```python
from build123d import *

# Parameters (mm, degrees)
F2_DEPTH = 25


with BuildPart() as f2:
    # F1 (on Top) → F2 (new body)
    with BuildSketch(Plane.XY):
        with BuildLine():
            Line((-1.828092, -48.106283), (0, -48.106283))
            Line((0, -48.106283), (1.828092, -48.106283))
            Line((1.828092, -48.106283), (4.154787, -40.719498))
            ThreePointArc((4.154787, -40.719498), (6.403006, -40.426987), (8.63158, -40.010444))
            Line((8.63158, -40.010444), (13.12704, -46.316705))
            Line((13.12704, -46.316705), (14.865659, -45.751794))
            Line((14.865659, -45.751794), (16.604278, -45.186882))
            Line((16.604278, -45.186882), (16.534454, -37.442644))
            ThreePointArc((16.534454, -37.442644), (18.582246, -36.469712), (20.573027, -35.384888))
            Line((20.573027, -35.384888), (26.797206, -39.993326))
            Line((26.797206, -39.993326), (28.276164, -38.9188))
            Line((28.276164, -38.9188), (29.755121, -37.844275))
            Line((29.755121, -37.844275), (27.295614, -30.500643))
            ThreePointArc((27.295614, -30.500643), (28.942527, -28.942527), (30.500643, -27.295614))
            Line((30.500643, -27.295614), (37.844275, -29.755121))
            Line((37.844275, -29.755121), (38.9188, -28.276164))
            Line((38.9188, -28.276164), (39.993326, -26.797206))
            Line((39.993326, -26.797206), (35.384888, -20.573027))
            ThreePointArc((35.384888, -20.573027), (36.469712, -18.582246), (37.442644, -16.534454))
            Line((37.442644, -16.534454), (45.186882, -16.604278))
            Line((45.186882, -16.604278), (45.751794, -14.865659))
            Line((45.751794, -14.865659), (46.316705, -13.12704))
            Line((46.316705, -13.12704), (40.010444, -8.63158))
            ThreePointArc((40.010444, -8.63158), (40.426987, -6.403006), (40.719498, -4.154787))
            Line((40.719498, -4.154787), (48.106283, -1.828092))
            Line((48.106283, -1.828092), (48.106283, 0))
            Line((48.106283, 0), (48.106283, 1.828092))
            Line((48.106283, 1.828092), (40.719498, 4.154787))
            ThreePointArc((40.719498, 4.154787), (40.426987, 6.403006), (40.010444, 8.63158))
            Line((40.010444, 8.63158), (46.316705, 13.12704))
            Line((46.316705, 13.12704), (45.751794, 14.865659))
            Line((45.751794, 14.865659), (45.186882, 16.604278))
            Line((45.186882, 16.604278), (37.442644, 16.534454))
            ThreePointArc((37.442644, 16.534454), (36.469712, 18.582246), (35.384888, 20.573027))
            Line((35.384888, 20.573027), (39.993326, 26.797206))
            Line((39.993326, 26.797206), (38.9188, 28.276164))
            Line((38.9188, 28.276164), (37.844275, 29.755121))
            Line((37.844275, 29.755121), (30.500643, 27.295614))
            ThreePointArc((30.500643, 27.295614), (28.942527, 28.942527), (27.295614, 30.500643))
            Line((27.295614, 30.500643), (29.755121, 37.844275))
            Line((29.755121, 37.844275), (28.276164, 38.9188))
            Line((28.276164, 38.9188), (26.797206, 39.993326))
            Line((26.797206, 39.993326), (20.573027, 35.384888))
            ThreePointArc((20.573027, 35.384888), (18.582246, 36.469712), (16.534454, 37.442644))
            Line((16.534454, 37.442644), (16.604278, 45.186882))
            Line((16.604278, 45.186882), (14.865659, 45.751794))
            Line((14.865659, 45.751794), (13.12704, 46.316705))
            Line((13.12704, 46.316705), (8.63158, 40.010444))
            ThreePointArc((8.63158, 40.010444), (6.403006, 40.426987), (4.154787, 40.719498))
            Line((4.154787, 40.719498), (1.828092, 48.106283))
            Line((1.828092, 48.106283), (0, 48.106283))
            Line((0, 48.106283), (-1.828092, 48.106283))
            Line((-1.828092, 48.106283), (-4.154787, 40.719498))
            ThreePointArc((-4.154787, 40.719498), (-6.403006, 40.426987), (-8.63158, 40.010444))
            Line((-8.63158, 40.010444), (-13.12704, 46.316705))
            Line((-13.12704, 46.316705), (-14.865659, 45.751794))
            Line((-14.865659, 45.751794), (-16.604278, 45.186882))
            Line((-16.604278, 45.186882), (-16.534454, 37.442644))
            ThreePointArc((-16.534454, 37.442644), (-18.582246, 36.469712), (-20.573027, 35.384888))
            Line((-20.573027, 35.384888), (-26.797206, 39.993326))
            Line((-26.797206, 39.993326), (-28.276164, 38.9188))
            Line((-28.276164, 38.9188), (-29.755121, 37.844275))
            Line((-29.755121, 37.844275), (-27.295614, 30.500643))
            ThreePointArc((-27.295614, 30.500643), (-28.942527, 28.942527), (-30.500643, 27.295614))
            Line((-30.500643, 27.295614), (-37.844275, 29.755121))
            Line((-37.844275, 29.755121), (-38.9188, 28.276164))
            Line((-38.9188, 28.276164), (-39.993326, 26.797206))
            Line((-39.993326, 26.797206), (-35.384888, 20.573027))
            ThreePointArc((-35.384888, 20.573027), (-36.469712, 18.582246), (-37.442644, 16.534454))
            Line((-37.442644, 16.534454), (-45.186882, 16.604278))
            Line((-45.186882, 16.604278), (-45.751794, 14.865659))
            Line((-45.751794, 14.865659), (-46.316705, 13.12704))
            Line((-46.316705, 13.12704), (-40.010444, 8.63158))
            ThreePointArc((-40.010444, 8.63158), (-40.426987, 6.403006), (-40.719498, 4.154787))
            Line((-40.719498, 4.154787), (-48.106283, 1.828092))
            Line((-48.106283, 1.828092), (-48.106283, 0))
            Line((-48.106283, 0), (-48.106283, -1.828092))
            Line((-48.106283, -1.828092), (-40.719498, -4.154787))
            ThreePointArc((-40.719498, -4.154787), (-40.426987, -6.403006), (-40.010444, -8.63158))
            Line((-40.010444, -8.63158), (-46.316705, -13.12704))
            Line((-46.316705, -13.12704), (-45.751794, -14.865659))
            Line((-45.751794, -14.865659), (-45.186882, -16.604278))
            Line((-45.186882, -16.604278), (-37.442644, -16.534454))
            ThreePointArc((-37.442644, -16.534454), (-36.469712, -18.582246), (-35.384888, -20.573027))
            Line((-35.384888, -20.573027), (-39.993326, -26.797206))
            Line((-39.993326, -26.797206), (-38.9188, -28.276164))
            Line((-38.9188, -28.276164), (-37.844275, -29.755121))
            Line((-37.844275, -29.755121), (-30.500643, -27.295614))
            ThreePointArc((-30.500643, -27.295614), (-28.942527, -28.942527), (-27.295614, -30.500643))
            Line((-27.295614, -30.500643), (-29.755121, -37.844275))
            Line((-29.755121, -37.844275), (-28.276164, -38.9188))
            Line((-28.276164, -38.9188), (-26.797206, -39.993326))
            Line((-26.797206, -39.993326), (-20.573027, -35.384888))
            ThreePointArc((-20.573027, -35.384888), (-18.582246, -36.469712), (-16.534454, -37.442644))
            Line((-16.534454, -37.442644), (-16.604278, -45.186882))
            Line((-16.604278, -45.186882), (-14.865659, -45.751794))
            Line((-14.865659, -45.751794), (-13.12704, -46.316705))
            Line((-13.12704, -46.316705), (-8.63158, -40.010444))
            ThreePointArc((-8.63158, -40.010444), (-6.403006, -40.426987), (-4.154787, -40.719498))
            Line((-4.154787, -40.719498), (-1.828092, -48.106283))
        make_face()
        with BuildLine():
            ThreePointArc((32.605994, 0), (23.05592, -23.05592), (0, -32.605994))
            ThreePointArc((0, -32.605994), (-23.05592, 23.05592), (32.605994, 0))
        make_face(mode=Mode.SUBTRACT)
    extrude(amount=F2_DEPTH)


solid = f2.part
```
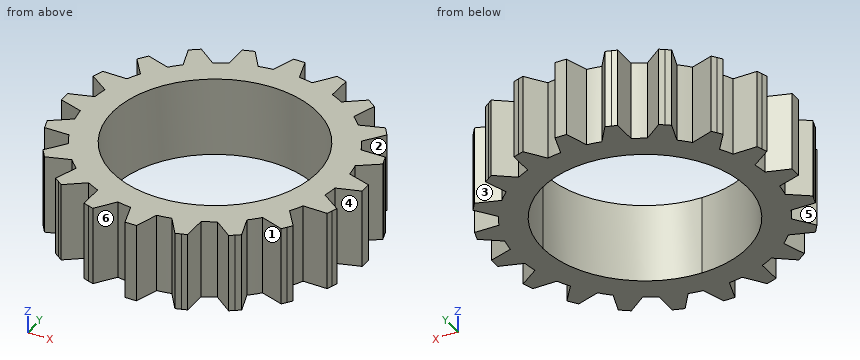
Geometry check sheet. Reference: the model listing, model coordinates, mm. Face numbers are marked on the shaded views. A direction names the side the tool comes from. Round coordinates to 2 decimals unless told otherwise and drop trailing zeros. Use a Markdown table: item, result.
(1) Scan lines: probe 1 along Y at (x, z) = (-43.5, 24.25); probe 2 along X at (y, z) = (-43, 4.5); probe 3 along Y at (x, z) = (-38, 16.5). Record each from-to range of solid material in increasing order.
Calculated:
| item | result |
|---|---|
| probe 1 | -16.59 to -11.12, -3.28 to 3.28, 11.12 to 16.59 |
| probe 2 | -16.58 to -10.76, -3.44 to 3.44, 10.76 to 16.58 |
| probe 3 | -29.54 to -24.11, -16.54 to 16.54, 24.11 to 29.54 |
(2) Go/stop test with flat-tipped pins: P1, Ø5, axis at x = -7.5, z = 12.5, coming from the -Y side; P2, Ø4, axis at x = 9.5, z = 4, coming from the +Y side; P3, Ø1.5, axis at y = 29.5, z = 6.5, coming from the +X side. Record where each tip stops, or that it passes through.
Calculated:
| item | result |
|---|---|
| P1 | y = -41.93 |
| P2 | y = 44.03 |
| P3 | x = 38.57 |
(3) Set-up check for the marked faces 1, 2 and 3: record each of +Z, -Z, +X, -X, +Y, -Y from which the full face is reachable in a straight line by a thin tool's end or side.
Calculated:
| item | result |
|---|---|
| face 1 | +Z, -Z, -Y |
| face 2 | +Z, -Z, +X |
| face 3 | +Z, -Z, +Y |
(4) Mould release check, pull along X, two halves, no side actions. Record for the marked faces 4, 5 and 6: released by +X, released by -X, zero draft, split by the parting line, or undercut.
Calculated:
| item | result |
|---|---|
| face 4 | released by +X |
| face 5 | released by -X |
| face 6 | undercut |
